Check sheet for the drawn part. Datum: minimum x, y, z corner. Units: mm. A direction names the side the tool comes from. Coordinates: 2 decimals unless noted, no trailing zeros. Write each loop counter-clockwise with the first axis right and the second up, starting at its lowest first coordinate (ties: lowest second). Pieces come first, ordered by that corner, then holes. Notation, with made-up numbers: (-13, -2) - (12, -2) arc R10 cw to (12, 2) - close; hole circle Ø3 at (48.5, -20.5). An arc over 180 degrees is marked (long way). Write each question's results on one line, items separated by ' | '.
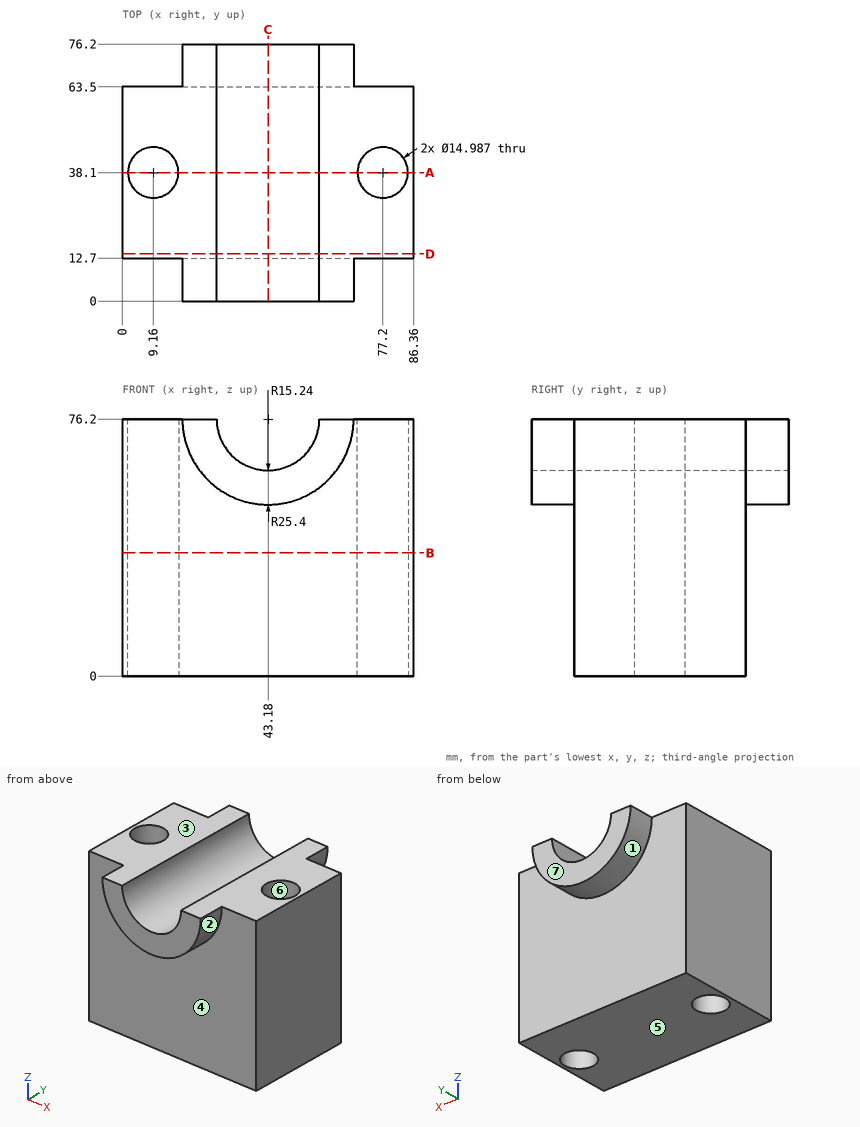
1. Sectioned sample at A-A (y = 38.1). Record the cut outline in (x, z).
Values follow:
outline: (0, 0) - (1.67, 0) - (1.67, 76.2) - (0, 76.2) - close; (16.65, 0) - (69.71, 0) - (69.71, 76.2) - (58.42, 76.2) arc R15.24 cw to (27.94, 76.2) - (16.65, 76.2) - close; (84.69, 0) - (86.36, 0) - (86.36, 76.2) - (84.69, 76.2) - close
2. Sectioned sample at D-D (y = 14). Record the cut outline in (x, z), then the cut area to 3 significant figures.
Values follow:
outline: (0, 0) - (86.36, 0) - (86.36, 76.2) - (58.42, 76.2) arc R15.24 cw to (27.94, 76.2) - (0, 76.2) - close | area: 6,220 mm^2
3. Go/stop test with flat-tipped pins: pin 1 (4 mm diameter, centred on y = 14, z = 45, fed in from -X); pin 2 (5 mm diameter, centred on x = 40.5, z = 8, fed in from -Y); pin 3 (9 mm diameter, centred on x = 9.16, y = 38.1, fed in from -Z). Record where each tip stops, or that it passes through.
Values follow:
pin 1: stops at x = 0 | pin 2: stops at y = 12.7 | pin 3: passes through
4. Sectioned sample at C-C (x = 43.18). Record the cut outline in (y, z), then the cut area to 3 significant figures.
Values follow:
outline: (0, 50.8) - (12.7, 50.8) - (12.7, 0) - (63.5, 0) - (63.5, 50.8) - (76.2, 50.8) - (76.2, 60.96) - (0, 60.96) - close | area: 3,350 mm^2
5. Sectioned sample at B-B (z = 36.5). Record the cut outline in (x, y).
Values follow:
outline: (0, 12.7) - (86.36, 12.7) - (86.36, 63.5) - (0, 63.5) - close; hole circle Ø14.99 at (9.16, 38.1); hole circle Ø14.99 at (77.2, 38.1)
6. Draft check along Y on the marked faces 4, 5, 6 and 7. Enter one of: pulls with the +Y half, pulls with the -Y half, needs draft (parallel to the pull), parting line crosses it, or undercut.
Values follow:
face 4: pulls with the -Y half | face 5: needs draft | face 6: undercut | face 7: pulls with the +Y half
7. Access from +Z, -Z, +X, -X, +Y, -Y to the whole of each face (thin tool, end or side, straight path). Record for the marked faces 1, 2 and 3.
Values follow:
face 1: -Z, +Y | face 2: -Z, -Y | face 3: +Z, +X, -X, +Y, -Y
8. Material ranges on L1, parallel to X at y = 38, z = 29; L2, parallel to Y at x = 27.5, z = 17.5; L3, parallel to X at y = 32.5, z = 21.5, recorded low to high. Write a range as [from, to].
Values follow:
L1: x = [0, 1.67], [16.65, 69.71], [84.69, 86.36] | L2: y = [12.7, 63.5] | L3: x = [0, 4.18], [14.14, 72.22], [82.18, 86.36]
